from build123d import *

# Parameters (mm, degrees)
F0_R      = 2.3
F1_DEPTH  = 25
F2_R      = 5
F2_R_2    = 5.3261161738
F3_DEPTH  = 5
F7_DEPTH  = 15.5
F9_R      = 2.3
F10_DEPTH = 38
F11_R     = 5
F12_DEPTH = 5.5


with BuildPart() as f1:
    # F0 (on Front) → F1 (new body)
    with BuildSketch(Plane.XZ):
        with BuildLine():
            ThreePointArc((18.5, -40), (19.5606601718, -39.5606601718), (20, -38.5))
            Line((20, -38.5), (20, 38.5))
            ThreePointArc((20, 38.5), (19.5606601718, 39.5606601718), (18.5, 40))
            Line((18.5, 40), (-18.5, 40))
            ThreePointArc((-18.5, 40), (-19.5606601718, 39.5606601718), (-20, 38.5))
            Line((-20, 38.5), (-20, -38.5))
            ThreePointArc((-20, -38.5), (-19.5606601718, -39.5606601718), (-18.5, -40))
            Line((-18.5, -40), (18.5, -40))
        make_face()
        with Locations((-10, -30)):
            Circle(F0_R, mode=Mode.SUBTRACT)
        with Locations((10, -30)):
            Circle(F0_R, mode=Mode.SUBTRACT)
        with Locations((-10, 30)):
            Circle(F0_R, mode=Mode.SUBTRACT)
        with Locations((10, 30)):
            Circle(F0_R, mode=Mode.SUBTRACT)
    extrude(amount=F1_DEPTH)

    # F2 (on face) → F3 (cut)
    with BuildSketch(Plane(origin=(0, 0, 0), x_dir=(-1, 0, 0), z_dir=(0, 1, 0))):
        with Locations((-10, 30)):
            Circle(F2_R)
        with Locations((10, 30)):
            Circle(F2_R)
        with Locations((10, -30)):
            Circle(F2_R_2)
        with Locations((-10, -30)):
            Circle(F2_R)
    extrude(amount=-F3_DEPTH, mode=Mode.SUBTRACT)

    # F6 (on offset) → F7 (cut, through all)
    with BuildSketch(Plane(origin=(0, 0, 0), x_dir=(0, -1, 0), z_dir=(-1, 0, 0))):
        with BuildLine():
            Line((15, -13), (25, -13))
            Line((25, -13), (25, 13))
            Line((25, 13), (15, 13))
            ThreePointArc((15, 13), (2, 0), (15, -13))
        make_face()
    extrude(amount=-F7_DEPTH, mode=Mode.SUBTRACT)

    # F9 (on face) → F10 (cut, through all)
    with BuildSketch(Plane(origin=(-20, 0, 0), x_dir=(0, -1, 0), z_dir=(-1, 0, 0))):
        with Locations((15, 0)):
            Circle(F9_R)
    extrude(amount=-F10_DEPTH, mode=Mode.SUBTRACT)

    # F11 (on face) → F12 (cut)
    with BuildSketch(Plane(origin=(-20, 0, 0), x_dir=(0, -1, 0), z_dir=(-1, 0, 0))):
        with Locations((15, 0)):
            Circle(F11_R)
    extrude(amount=-F12_DEPTH, mode=Mode.SUBTRACT)


solid = f1.part
Source: CAD feature listing. Evaluate the final solid. Frame: model axes, mm. A direction names the side the tool comes from. Coordinates: 2 decimals unless noted, no trailing zeros. Order: outer loops, then holes, each group sorted by start corner. A loop starts at its lowest first (then second) coordinate and runs counter-clockwise, first axis right, second up. Notation, with made-up numbers: M 22,76 L 37,76 A26 ccw 37,102 Z; hole C -40,36 d7. An arc over 180 degrees is marked long. Write each question's results on one line, items separated by ' | '. Start each with the question number.
1. Material intervals for L1, parallel to Z at x = -10, y = -2.75; L2, parallel to Z at x = 10, y = -17.75; L3, parallel to X at y = -16.5, z = -30, sorted ascending.
2. Reachability of faces 1 (the face through (-11.1, -5, -32.3)), 2 (the face through (-17.29, -19.77, 1.5)), 3 (the face through (-12.298, -14.86, -29.899)), 4 (the face through (0, -13, 3)), 5 (the face through (-19.57, -12.32, -39.55)) from +Z, -Z, +X, -X, +Y, -Y: full face, straight path, thin tool, end or side. Return the list, or none.
3. Section D-D, the plane y = -16. Return the cut outline in (x, z), then the cut area to 3 significant figures.
4. Section B-B, the plane x = 10. Return the cut outline in (y, z).
5. Section A-A, the plane z = -30. Return the cut outline in (x, y), then the cut area to 3 significant figures.
6. Section C-C, the plane z = 0. Return the cut outline in (x, y).
7. Pin query (flat end, axial travel): pin 1 (6 mm diameter, centred on x = 10, z = 30, fed in from +Y); pin 2 (2.5 mm diameter, centred on y = -15.5, z = -1, fed in from -X). Return the tip coordinate at first contact, or that it passes through.
8. Draft query along X for faces 6 (the face through (16.732, -17.194, 0.691)), 7 (the face through (-14.619, -2.465, 28.085)), 8 (the face through (19.57, -12.32, 39.55)). Return one class per face: +X half, -X half, draft (parallel to the pull), parting line (faces both ways), or undercut.
Solution:
1) L1: -40 to -35.33, -24.67 to 25, 35 to 40 | L2: -40 to -32.3, -27.7 to -13, 13 to 27.7, 32.3 to 40 | L3: -20 to -12.3, -7.7 to 7.7, 12.3 to 20
2) face 1: +Y | face 2: -X | face 3: +Y, -Y | face 4: -Y | face 5: -Z, -X, +Y, -Y
3) outline: M -20,-38.5 A1.5 ccw -18.5,-40 L 18.5,-40 A1.5 ccw 20,-38.5 L 20,38.5 A1.5 ccw 18.5,40 L -18.5,40 A1.5 ccw -20,38.5 L -20,4.9 L -14.5,4.9 L -14.5,2.07 L 0,2.07 L 0,13 L 15.5,13 L 15.5,2.07 L 18,2.07 L 18,-2.07 L 15.5,-2.07 L 15.5,-13 L 0,-13 L 0,-2.07 L -14.5,-2.07 L -14.5,-4.9 L -20,-4.9 Z; hole C -10,-30 d4.6; hole C -10,30 d4.6; hole C 10,-30 d4.6; hole C 10,30 d4.6 | area: 2,600 mm²
4) outline: M -25,-40 L 0,-40 L 0,-35 L -5,-35 L -5,-32.3 L -25,-32.3 Z; M -25,-27.7 L -5,-27.7 L -5,-25 L 0,-25 L 0,25 L -5,25 L -5,27.7 L -25,27.7 L -25,13 L -15,13 A13 cw -15,-13 L -25,-13 Z; M -25,32.3 L -5,32.3 L -5,35 L 0,35 L 0,40 L -25,40 Z
5) outline: M -20,-25 L -12.3,-25 L -12.3,-5 L -15.33,-5 L -15.33,0 L -20,0 Z; M -7.7,-25 L 7.7,-25 L 7.7,-5 L 5,-5 L 5,0 L -4.67,0 L -4.67,-5 L -7.7,-5 Z; M 12.3,-25 L 20,-25 L 20,0 L 15,0 L 15,-5 L 12.3,-5 Z | area: 713 mm²
6) outline: M -20,-25 L 0,-25 L 0,-17.3 L -14.5,-17.3 L -14.5,-20 L -20,-20 Z; M -20,-10 L -14.5,-10 L -14.5,-12.7 L 0,-12.7 L 0,-2 L 15.5,-2 L 15.5,-12.7 L 18,-12.7 L 18,-17.3 L 15.5,-17.3 L 15.5,-25 L 20,-25 L 20,0 L -20,0 Z
7) pin 1: y = -5 | pin 2: x = -14.5
8) face 6: draft | face 7: undercut | face 8: +X half
